Check sheet for the drawn part. Datum: minimum x, y, z corner. Units: mm. A direction names the side the tool comes from. Give positions to 0.01 mm unless a question says otherwise; leave off trailing zeros. Loops run counter-clockwise (first coordinate to the right, second up) from the corner with the lowest first, then second, coordinate; pieces in that order, holes last. Notation, with made-up numbers: (-12.5, -7) - (28.5, -7) arc R33 ccw to (28.5, 31) - close; hole circle Ø7 at (78, 51). An arc over 180 degrees is marked (long way). One line per item, written item: value. Start each with the question number.
1. Access from +Z, -Z, +X, -X, +Y, -Y to the whole of each face (thin tool, end or side, straight path). Record for the marked faces 1 and 2.
2. Gauge pin test, flat end, axial feed: pin 1 (0.6 mm diameter, centred on x = 3.5, z = 7, fed in from -Y). Record the tip position at first contact, or that the pin passes through.
3. Scan lines: L1, parallel to Z at x = 3.8, y = 4.85; L2, parallel to Z at x = 1.7, y = 2.7; L3, parallel to X at y = 2.85, z = 5.5. Record each from-to range of solid material in increasing order. Write a range as [from, to].
4. Sectioned sample at A-A (x = 2.75). Record the cut outline in (y, z) (3 decimals).
5. Sectioned sample at B-B (y = 2.75). Record the cut outline in (x, z) (3 decimals), plus the area to 3 significant figures.
6. Sectioned sample at D-D (y = 2). Record the cut outline in (x, z).
7. Sectioned sample at C-C (z = 5.5). Record the cut outline in (x, y), plus the area to 3 significant figures.
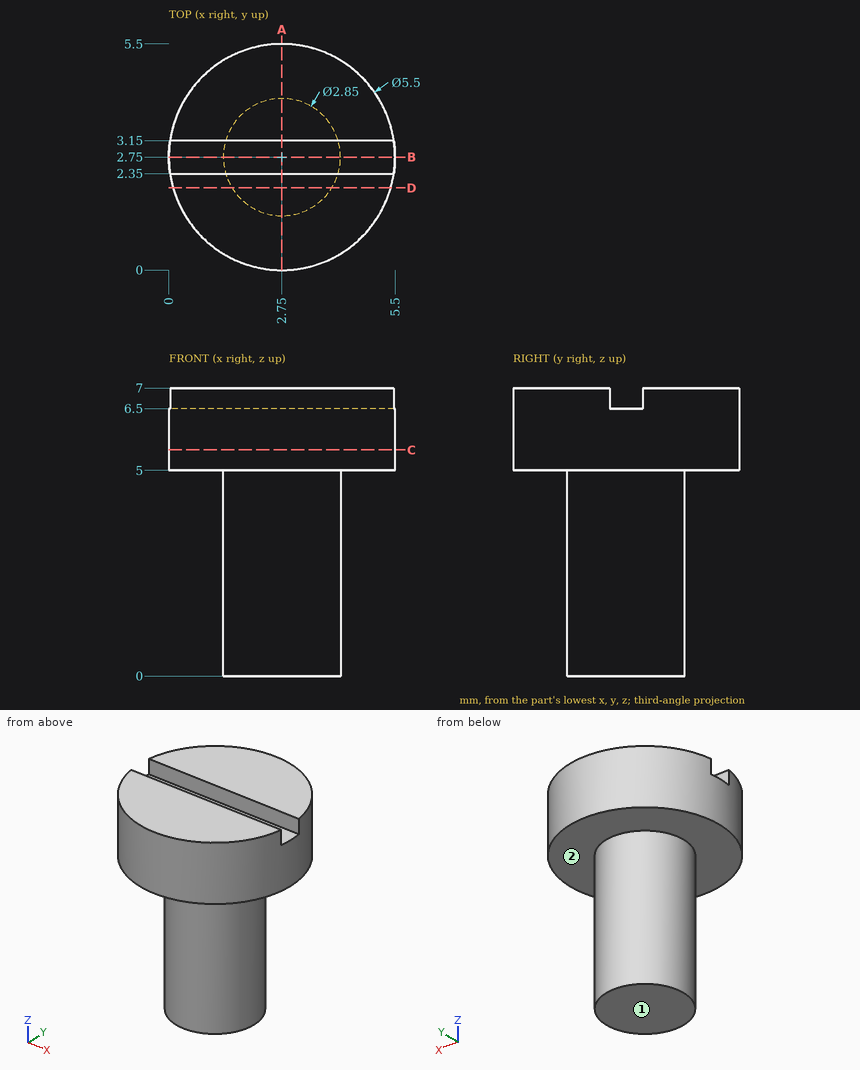
Results are:
1. face 1: -Z, +X, -X, +Y, -Y
1. face 2: -Z
2. pin 1: stops at y = 0.04
3. L1: z = [5, 7]
3. L2: z = [0, 6.5]
3. L3: x = [0, 5.5]
4. outline: (0, 5) - (1.325, 5) - (1.325, 0) - (4.175, 0) - (4.175, 5) - (5.5, 5) - (5.5, 7) - (3.15, 7) - (3.15, 6.5) - (2.35, 6.5) - (2.35, 7) - (0, 7) - close
5. outline: (0, 5) - (1.325, 5) - (1.325, 0) - (4.175, 0) - (4.175, 5) - (5.5, 5) - (5.5, 6.5) - (0, 6.5) - close
5. area: 22.5 mm^2
6. outline: (0.1, 5) - (1.54, 5) - (1.54, 0) - (3.96, 0) - (3.96, 5) - (5.4, 5) - (5.4, 7) - (0.1, 7) - close
7. outline: circle Ø5.5 at (2.75, 2.75)
7. area: 23.8 mm^2
